from build123d import *

# Parameters (mm, degrees)
ESQUISSE1_R               = 110
BOSS_EXTRU_1_DEPTH        = 3
D_GAGEMENT_M61_AT_2_COUNT = 2
D_GAGEMENT_M61_AT_2_PITCH = 127.279220614
D_GAGEMENT_M61_AT_3_COUNT = 2
D_GAGEMENT_M61_AT_3_PITCH = 127.279220614
D_GAGEMENT_M61_AT_4_COUNT = 2
D_GAGEMENT_M61_AT_4_PITCH = 180
ESQUISSE2_W               = 30
ESQUISSE2_H               = 50
ESQUISSE2_W_2             = 50
ESQUISSE2_H_2             = 30
ENL_V_MAT_EXTRU_1_DEPTH   = 10


with BuildPart() as part:
    # Esquisse1 → Boss.-Extru.1 (new body)
    with BuildSketch(Plane.XY):
        Circle(ESQUISSE1_R)
    extrude(amount=BOSS_EXTRU_1_DEPTH)

    # Esquisse4 → Dégagement M61 (revolve, cut)
    with BuildSketch(Plane(origin=(-63.639610307, 63.639610307, 3), x_dir=(0, -1, 0), z_dir=(1, 0, 0))):
        Polygon((0, 0), (0, 3), (3.3, 3), (3.3, 0.025), (3.325, 0), align=None)
    d_gagement_m61 = revolve(axis=Axis((-63.639610307, 63.639610307, 9.35), (0, 0, -1)), mode=Mode.SUBTRACT)

    # Dégagement M61 at 2: Dégagement M61 ×2
    with Locations(*[(i * D_GAGEMENT_M61_AT_2_PITCH, 0, 0) for i in range(1, D_GAGEMENT_M61_AT_2_COUNT)]):
        add(d_gagement_m61, mode=Mode.SUBTRACT)

    # Dégagement M61 at 3: Dégagement M61 ×2
    with Locations(*[(0, -i * D_GAGEMENT_M61_AT_3_PITCH, 0) for i in range(1, D_GAGEMENT_M61_AT_3_COUNT)]):
        add(d_gagement_m61, mode=Mode.SUBTRACT)

    # Dégagement M61 at 4: Dégagement M61 ×2
    with Locations(*[Vector(0.7071067811865517, -0.7071067811865435, 0) * (i * D_GAGEMENT_M61_AT_4_PITCH) for i in range(1, D_GAGEMENT_M61_AT_4_COUNT)]):
        add(d_gagement_m61, mode=Mode.SUBTRACT)

    # Esquisse2 → Enlèv. mat.-Extru.1 (cut)
    with BuildSketch(Plane(origin=(0, 0, 0), x_dir=(-1, 0, 0), z_dir=(0, 0, -1))):
        with Locations((95, 0)):
            Rectangle(ESQUISSE2_W, ESQUISSE2_H)
        with Locations((-95, 0)):
            Rectangle(ESQUISSE2_W, ESQUISSE2_H)
        with Locations((0, -95)):
            Rectangle(ESQUISSE2_W_2, ESQUISSE2_H_2)
        with Locations((0, 95)):
            Rectangle(ESQUISSE2_W_2, ESQUISSE2_H_2)
    extrude(amount=-ENL_V_MAT_EXTRU_1_DEPTH, mode=Mode.SUBTRACT)


solid = part.part
Geometry check sheet. Reference: the model listing, model coordinates, mm. Round coordinates to 2 decimals unless told otherwise and drop trailing zeros. Order: outer loops, then holes, each group sorted by start corner. A loop starts at its lowest first (then second) coordinate and runs counter-clockwise, first axis right, second up. Notation, with made-up numbers: M 71,67.25 L 98,67.25 A21 cw 98,75.25 Z; hole C -16,-28 d9. An arc over 180 degrees is marked long. Answer in a Markdown table with one row per item.
(1) Sectioned sample at A-A, the plane y = 83. Record the cut outline in (x, z), and give its area (3 significant figures).
Responses:
| item | result |
|---|---|
| outline | M -72.19,0 L -25,0 L -25,3 L -72.19,3 Z; M 25,0 L 72.19,0 L 72.19,3 L 25,3 Z |
| area | 283 mm² |
(2) Sectioned sample at C-C, the plane x = -13. Record the cut outline in (y, z).
Responses:
| item | result |
|---|---|
| outline | M -80,0 L 80,0 L 80,3 L -80,3 Z |
(3) Draft check along X on faces 1 (the face through (-77.174, 78.385, 1.479)), 2 (the face through (-1, 1, 0)), 3 (the face through (-63.785, -60.343, 1.508)), 4 (the face through (78.385, 77.174, 1.479)). Enter one of: released by +X, released by -X, zero draft, split by the parting line, or undercut.
Responses:
| item | result |
|---|---|
| face 1 | released by -X |
| face 2 | zero draft |
| face 3 | undercut |
| face 4 | released by +X |
(4) Sectioned sample at B-B, the plane z = 2.4. Record the cut outline in (x, y), and give its area (3 significant figures).
Responses:
| item | result |
|---|---|
| outline | M -107.12,-25 A110 ccw -25,-107.12 L -25,-80 L 25,-80 L 25,-107.12 A110 ccw 107.12,-25 L 80,-25 L 80,25 L 107.12,25 A110 ccw 25,107.12 L 25,80 L -25,80 L -25,107.12 A110 ccw -107.12,25 L -80,25 L -80,-25 Z; hole C -63.64,-63.64 d6.6; hole C -63.64,63.64 d6.6; hole C 63.64,-63.64 d6.6; hole C 63.64,63.64 d6.6 |
| area | 32,100 mm² |
(5) Scan lines: probe 1 along Y at (x, z) = (65, 1.9); probe 2 along Y at (x, z) = (61, 1.45); probe 3 along Y at (x, z) = (84, 0.95). Record each from-to range of solid material in increasing order. Write a range as from..to.
Responses:
| item | result |
|---|---|
| probe 1 | y = -88.74..-66.65, -60.63..60.63, 66.65..88.74 |
| probe 2 | y = -91.54..-65.62, -61.66..61.66, 65.62..91.54 |
| probe 3 | y = -71.02..-25, 25..71.02 |
(6) Go/stop test with flat-tipped pins: P1, Ø0.9, axis at x = 98, z = 1.5, coming from the +Y side; P2, Ø1.5, axis at y = -94, z = 1, coming from the +X side; P3, Ø0.9, axis at y = 93, z = 1.5, coming from the +X side. Record where each tip stops, or that it passes through.
Responses:
| item | result |
|---|---|
| P1 | stops at y = 50.83 |
| P2 | stops at x = 58.35 |
| P3 | stops at x = 59.45 |
